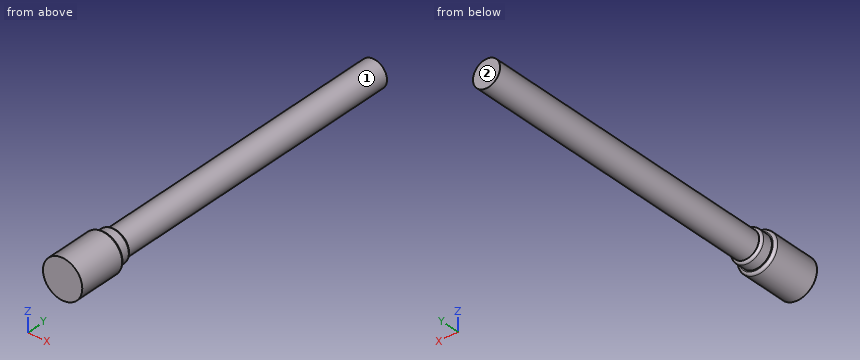
```python
from build123d import *

# Parameters (mm, degrees)
F0_R     = 11
F1_DEPTH = 250
F2_R     = 13
F2_R_2   = 11
F3_DEPTH = 10
F4_R     = 1.99999
F5_R     = 16
F5_R_2   = 13
F6_DEPTH = 40
F7_R     = 2


# Not quite as in the source:
# - a fillet or chamfer is up to 0.001 mm smaller than in the source, because OpenCascade refuses the exact size


with BuildPart() as f1:
    # F0 (on Front) → F1 (new body)
    with BuildSketch(Plane.XZ):
        Circle(F0_R)
    extrude(amount=F1_DEPTH)

    # F2 (on face) → F3 (join)
    with BuildSketch(Plane.XZ.offset(250)):
        Circle(F2_R)
        Circle(F2_R_2, mode=Mode.SUBTRACT)
        Circle(F2_R_2)
    extrude(amount=F3_DEPTH)

    # F4 (radius 2 in the source; OpenCascade refuses exactly that, so slightly less here)
    f4_edges = [f1.edges().sort_by_distance(p)[0] for p in [
        (-13, -250, 0),
    ]]
    fillet(f4_edges, radius=F4_R)

    # F5 (on face) → F6 (join)
    with BuildSketch(Plane.XZ.offset(260)):
        Circle(F5_R)
        Circle(F5_R_2, mode=Mode.SUBTRACT)
        Circle(F5_R_2)
    extrude(amount=F6_DEPTH)

    # F7
    f7_edges = [f1.edges().sort_by_distance(p)[0] for p in [
        (-16, -260, 0),
    ]]
    fillet(f7_edges, radius=F7_R)


solid = f1.part
```
Source: CAD feature listing. Evaluate the final solid. Frame: model axes, mm. Face numbers are marked on the shaded views. A direction names the side the tool comes from. Coordinates: 2 decimals unless noted, no trailing zeros. Order: outer loops, then holes, each group sorted by start corner. A loop starts at its lowest first (then second) coordinate and runs counter-clockwise, first axis right, second up. Notation, with made-up numbers: M -26.5,-2 L -10.5,-2 A20 cw -10.5,12 Z; hole C 51,72 d4. An arc over 180 degrees is marked long. Write each question's results on one line, items separated by ' | '. Start each with the question number.
1) Contact query for flat-ended pins moving along their axis: pin 1 Ø5 at (y, z) = (-92, -8.5) entering from +X; pin 2 Ø1 at (y, z) = (-232, 12) entering from +X; pin 3 Ø1.5 at (y, z) = (-43.5, 9.5) entering from -X; pin 4 Ø3 at (x, y) = (0, -128.5) entering from +Z. Output: stop coordinate, or through.
2) Line query: line 1 (Y direction, x = 13.5, z = -2); line 2 (X direction, y = -196, z = -1); line 3 (Y direction, x = 6.5, z = 9). Output: solid intervals per line, ascending. Write a range as from..to.
3) Access query for the marked faces 1 and 2. Directions: +Z, -Z, +X, -X, +Y, -Y. A direction counts if a zero-diameter tool reaches every point of the face in a straight line with its end or side. Return the directions, or none.
4) Section query C-C (y = -190.5). Return the cut outline in (x, z).
Answers:
1) pin 1: stops at x = 9.22 | pin 2: passes through | pin 3: stops at x = -6.67 | pin 4: stops at z = 11
2) line 1: y = -300..-260 | line 2: x = -10.95..10.95 | line 3: y = -300..-250
3) face 1: +Y | face 2: +Z, -Z, +X, -X, +Y
4) outline: C 0,0 d22
